The figure shows three views and two pictorial views of one solid part (mm, origin at its lowest corner). Answer the questions. Coordinates: 2 decimals unless noted, no trailing zeros. Write each loop counter-clockwise with the first axis right and the second up, starting at its lowest first coordinate (ties: lowest second). Pieces come first, ordered by that corner, then holes.
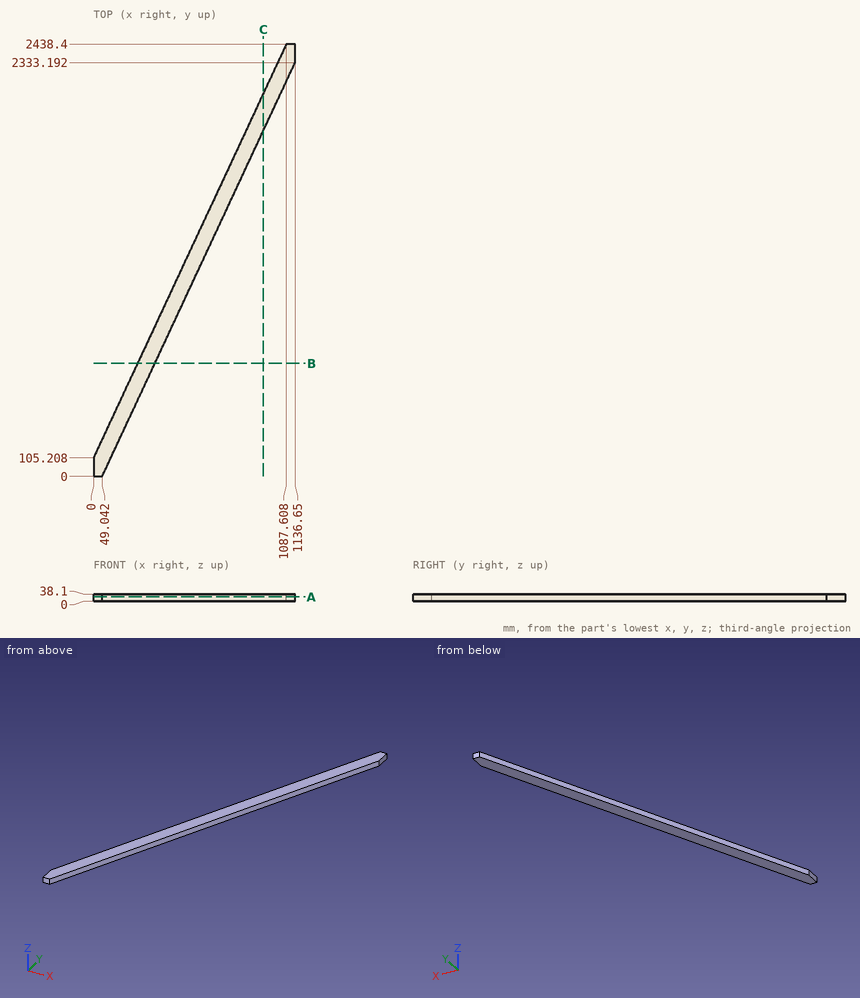
Q1. The part is cut by section A-A, the plane z = 24. Write down the section's boundary in (x, y), then the cut area to 3 significant figures.
Answers below:
outline: (0, 0) - (49.04, 0) - (1136.65, 2333.19) - (1136.65, 2438.4) - (1087.61, 2438.4) - (0, 105.21) - close
area: 234,000 mm2
Q2. Find the intervals of material crossed by probe 1 along Y at (x, z) = (177.5, 25.5) (1 decimal); probe 2 along Y at (x, z) = (261.5, 11.5) (1 decimal); probe 3 along X at (y, z) = (1458, 36), in increasing order.
Answers below:
probe 1: y = 275.6 to 486
probe 2: y = 455.8 to 666.2
probe 3: x = 630.6 to 728.68
Q3. The part is cut by section B-B, the plane y = 637. Write down the section's boundary in (x, z), then the cut area to 3 significant figures.
Answers below:
outline: (247.89, 0) - (345.98, 0) - (345.98, 38.1) - (247.89, 38.1) - close
area: 3,740 mm2
Q4. The part is cut by section C-C, the plane x = 958.5. Write down the section's boundary in (y, z).
Answers below:
outline: (1951.02, 0) - (2161.43, 0) - (2161.43, 38.1) - (1951.02, 38.1) - close
Q5. Given pin 1 (1.5 mm diameter, centred on x = 168.5, z = 27.5, fed in from -Y); pin 2 (1 mm diameter, centred on y = 1066.5, z = 31, fed in from -X); pin 3 (6 mm diameter, centred on y = 1608, z = 24, fed in from +X), each flat-ended and moving along its own axis, determine where each tip first touches the part or whether it passes through.
Answers below:
pin 1: stops at y = 254.66
pin 2: stops at x = 447.87
pin 3: stops at x = 800
